from build123d import *

# Parameters (mm, degrees)
F0_W      = 105.5624
F0_H      = 50.8
F1_DEPTH  = 198.4375
F2_W      = 105.5624
F2_H      = 38.1
F3_DEPTH  = 15.875
F5_DEPTH  = 182.5635
F6_W      = 105.5624
F6_H      = 38.1
F7_DEPTH  = 17.4498
F9_DEPTH  = 25.4
F10_R     = 1.27
F11_DEPTH = 182.5635


with BuildPart() as f1:
    # F0 (on Front) → F1 (new body)
    with BuildSketch(Plane.XZ):
        with Locations((52.7812, 25.4)):
            Rectangle(F0_W, F0_H)
    extrude(amount=-F1_DEPTH)

    # F2 (on face) → F3 (cut)
    with BuildSketch(Plane.XZ):
        with Locations((52.7812, 31.75)):
            Rectangle(F2_W, F2_H)
    extrude(amount=-F3_DEPTH, mode=Mode.SUBTRACT)

    # F4 (on face) → F5 (cut, through all)
    with BuildSketch(Plane.XZ.offset(-15.875)):
        Polygon((29.765625, 50.8), (16.933333, 50.8), (16.933333, 39.6875), (11.244792, 39.6875), (11.244792, 32.0675), (35.454167, 32.0675), (35.454167, 39.290625), (29.765625, 39.290625), align=None)
        Polygon((105.5624, 50.8), (47.625, 50.8), (47.625, 25.4), (80.1624, 25.4), (80.1624, 41.275), (105.5624, 41.275), align=None)
    extrude(amount=-F5_DEPTH, mode=Mode.SUBTRACT)

    # F6 (on face) → F7 (cut)
    with BuildSketch(Plane(origin=(0, 198.4375, 0), x_dir=(-1, 0, 0), z_dir=(0, 1, 0))):
        with Locations((-52.7812, 31.75)):
            Rectangle(F6_W, F6_H)
    extrude(amount=-F7_DEPTH, mode=Mode.SUBTRACT)

    # F8 (on face) → F9 (cut, through all)
    with BuildSketch(Plane.YZ.offset(105.5624)):
        with BuildLine():
            Line((30.16885, 33.3375), (34.93135, 33.3375))
            ThreePointArc((34.93135, 33.3375), (30.16885, 38.1), (25.40635, 33.3375))
            Line((25.40635, 33.3375), (30.16885, 33.3375))
        make_face()
        with BuildLine():
            ThreePointArc((25.40635, 33.3375), (30.16885, 28.575), (34.93135, 33.3375))
            Line((34.93135, 33.3375), (30.16885, 33.3375))
            Line((30.16885, 33.3375), (25.40635, 33.3375))
        make_face()
        with BuildLine():
            ThreePointArc((171.45635, 33.3375), (166.69385, 38.1), (161.93135, 33.3375))
            Line((161.93135, 33.3375), (166.69385, 33.3375))
            Line((166.69385, 33.3375), (171.45635, 33.3375))
        make_face()
        with BuildLine():
            Line((166.69385, 33.3375), (161.93135, 33.3375))
            ThreePointArc((161.93135, 33.3375), (166.69385, 28.575), (171.45635, 33.3375))
            Line((171.45635, 33.3375), (166.69385, 33.3375))
        make_face()
        with BuildLine():
            ThreePointArc((151.952779, 33.3375), (147.190279, 38.1), (142.427779, 33.3375))
            Line((142.427779, 33.3375), (147.190279, 33.3375))
            Line((147.190279, 33.3375), (151.952779, 33.3375))
        make_face()
        with BuildLine():
            Line((147.190279, 33.3375), (142.427779, 33.3375))
            ThreePointArc((142.427779, 33.3375), (147.190279, 28.575), (151.952779, 33.3375))
            Line((151.952779, 33.3375), (147.190279, 33.3375))
        make_face()
        with BuildLine():
            ThreePointArc((132.449207, 33.3375), (127.686707, 38.1), (122.924207, 33.3375))
            Line((122.924207, 33.3375), (127.686707, 33.3375))
            Line((127.686707, 33.3375), (132.449207, 33.3375))
        make_face()
        with BuildLine():
            Line((127.686707, 33.3375), (122.924207, 33.3375))
            ThreePointArc((122.924207, 33.3375), (127.686707, 28.575), (132.449207, 33.3375))
            Line((132.449207, 33.3375), (127.686707, 33.3375))
        make_face()
        with BuildLine():
            ThreePointArc((112.945636, 33.3375), (108.183136, 38.1), (103.420636, 33.3375))
            Line((103.420636, 33.3375), (108.183136, 33.3375))
            Line((108.183136, 33.3375), (112.945636, 33.3375))
        make_face()
        with BuildLine():
            Line((108.183136, 33.3375), (103.420636, 33.3375))
            ThreePointArc((103.420636, 33.3375), (108.183136, 28.575), (112.945636, 33.3375))
            Line((112.945636, 33.3375), (108.183136, 33.3375))
        make_face()
        with BuildLine():
            ThreePointArc((93.442064, 33.3375), (88.679564, 38.1), (83.917064, 33.3375))
            Line((83.917064, 33.3375), (88.679564, 33.3375))
            Line((88.679564, 33.3375), (93.442064, 33.3375))
        make_face()
        with BuildLine():
            Line((88.679564, 33.3375), (83.917064, 33.3375))
            ThreePointArc((83.917064, 33.3375), (88.679564, 28.575), (93.442064, 33.3375))
            Line((93.442064, 33.3375), (88.679564, 33.3375))
        make_face()
        with BuildLine():
            ThreePointArc((73.938493, 33.3375), (69.175993, 38.1), (64.413493, 33.3375))
            Line((64.413493, 33.3375), (69.175993, 33.3375))
            Line((69.175993, 33.3375), (73.938493, 33.3375))
        make_face()
        with BuildLine():
            Line((69.175993, 33.3375), (64.413493, 33.3375))
            ThreePointArc((64.413493, 33.3375), (69.175993, 28.575), (73.938493, 33.3375))
            Line((73.938493, 33.3375), (69.175993, 33.3375))
        make_face()
        with BuildLine():
            ThreePointArc((54.434921, 33.3375), (49.672421, 38.1), (44.909921, 33.3375))
            Line((44.909921, 33.3375), (49.672421, 33.3375))
            Line((49.672421, 33.3375), (54.434921, 33.3375))
        make_face()
        with BuildLine():
            Line((49.672421, 33.3375), (44.909921, 33.3375))
            ThreePointArc((44.909921, 33.3375), (49.672421, 28.575), (54.434921, 33.3375))
            Line((54.434921, 33.3375), (49.672421, 33.3375))
        make_face()
    extrude(amount=-F9_DEPTH, mode=Mode.SUBTRACT)

    # F10 (on face) → F11 (cut, through all)
    with BuildSketch(Plane.XZ.offset(-15.875)):
        with Locations((47.625, 25.4)):
            Circle(F10_R)
    extrude(amount=-F11_DEPTH, mode=Mode.SUBTRACT)


solid = f1.part
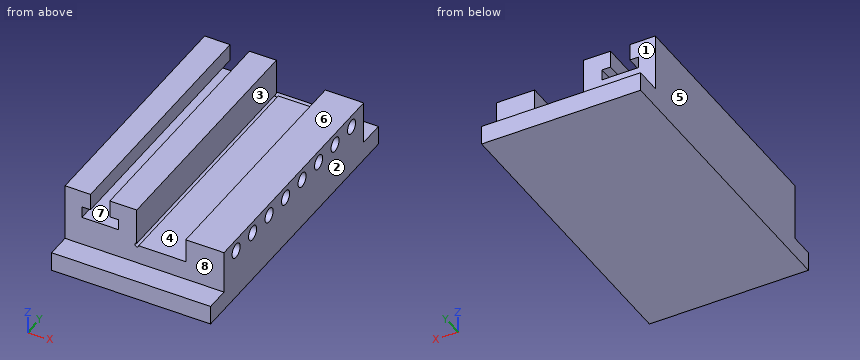
Source: CAD feature listing. Evaluate the final solid. Frame: model axes, mm. Face numbers are marked on the shaded views. A direction names the side the tool comes from. Coordinates: 2 decimals unless noted, no trailing zeros. Loops run counter-clockwise (first coordinate to the right, second up) from the corner with the lowest first, then second, coordinate; pieces in that order, holes last. Notation, with made-up numbers: (47.5, 61.25) - (67.5, 61.25) arc R19 ccw to (67.5, 87.25) - close; hole circle Ø1 at (89.5, -1). An arc over 180 degrees is marked (long way). One line per item, written item: value. Start each with the question number.
1. Section D-D (y = 22). Return the cut outline in (x, z) (1 decimal), and give its area (3 significant figures).
2. Section A-A (z = 45.5). Return the cut outline in (x, y) (3 decimals), and give its area (3 significant figures).
3. Set-up query: the marked faces 5, 6, 7 and 8. Return all of +Z, -Z, +X, -X, +Y, -Y with unobstructed straight access to the full face (end or side cutting, diameter ignored); none if empty.
4. Section C-C (y = 125.5). Return the cut outline in (x, z) (1 decimal).
5. Contact query for flat-ended pins moving along their axis: P1, Ø12.5, axis at x = 90, y = 117, coming from the +Z side (3 decimals); P2, Ø12, axis at x = 80, z = 32, coming from the +Y side; P3, Ø5, axis at x = 35.5, y = 7, coming from the +Z side. Output: stop coordinate, or through.
6. Ray query, L1, parallel to X at y = 85.5, z = 49 (3 decimals); L2, parallel to X at y = 103, z = 32 (3 decimals); L3, parallel to Z at x = 99.5, y = 167 (3 decimals). Return the intervals inside material, ascending.
7. Mould query, pull axis X, two halves, no side actions, for the marked faces 1, 2, 3 and 4. Classes: pulls with the +X half, pulls with the -X half, needs draft (parallel to the pull), parting line crosses it, or undercut.
8. Section B-B (x = 24). Return the cut outline in (y, z) (1 decimal), and give its area (3 significant figures).
Verdict:
1. outline: (0, 0) - (105.6, 0) - (105.6, 41.3) - (80.2, 41.3) - (80.2, 25.4) - (48.9, 25.4) arc R1.3 cw (long way) to (47.6, 26.7) - (47.6, 50.8) - (29.8, 50.8) - (29.8, 39.3) - (35.5, 39.3) - (35.5, 32.1) - (11.2, 32.1) - (11.2, 39.7) - (16.9, 39.7) - (16.9, 50.8) - (0, 50.8) - close
1. area: 3,970 mm2
2. outline: (0, 15.875) - (16.933, 15.875) - (16.933, 180.988) - (0, 180.988) - close; (29.766, 15.875) - (47.625, 15.875) - (47.625, 180.988) - (29.766, 180.988) - close
2. area: 5,740 mm2
3. face 5: +Z, -Z, -X, +Y, -Y
3. face 6: +Z, +X, +Y, -Y
3. face 7: +Y, -Y
3. face 8: +Z, +X, -X, -Y
4. outline: (0, 0) - (105.6, 0) - (105.6, 29.1) - (80.2, 29.1) - (80.2, 25.4) - (48.9, 25.4) arc R1.3 cw (long way) to (47.6, 26.7) - (47.6, 50.8) - (29.8, 50.8) - (29.8, 39.3) - (35.5, 39.3) - (35.5, 32.1) - (11.2, 32.1) - (11.2, 39.7) - (16.9, 39.7) - (16.9, 50.8) - (0, 50.8) - close; (80.2, 37.6) - (105.6, 37.6) - (105.6, 41.3) - (80.2, 41.3) - close
5. P1: stops at z = 41.275
5. P2: stops at y = 180.99
5. P3: stops at z = 12.7
6. L1: x = 0 to 16.933, 29.766 to 47.625
6. L2: x = 0 to 47.625, 80.162 to 105.562
6. L3: z = 0 to 28.585, 38.09 to 41.275
7. face 1: needs draft
7. face 2: pulls with the +X half
7. face 3: undercut
7. face 4: undercut
8. outline: (0, 0) - (198.4, 0) - (198.4, 12.7) - (181, 12.7) - (181, 32.1) - (15.9, 32.1) - (15.9, 12.7) - (0, 12.7) - close
8. area: 5,720 mm2
